```python
from build123d import *

# Parameters (mm, degrees)
F1_DEPTH = 25.4


with BuildPart() as f1:
    # F0 (on Front) → F1 (new body)
    with BuildSketch(Plane.XZ):
        Polygon((37.505187, 36.036089), (-59.895307, -2.682783), (38.255867, -41.096099), (18.550564, -2.999177), align=None)
        Polygon((5.644079, -12.203965), (-13.873555, -4.697184), (5.034152, -10.421105), align=None, mode=Mode.SUBTRACT)
        Polygon((11.606792, -2.682783), (26.432687, -31.33728), (-46.783395, -2.682783), (24.93133, 25.526594), (13.858826, 2.0679), (11.419123, 2.0679), (12.732809, 13.328073), (-28.366823, -2.682783), (13.1488, -18.930706), (7.523733, -8.055575), (-15.980633, -2.682783), align=None, mode=Mode.SUBTRACT)
        Polygon((6.774401, 3.053483), (-3.437838, 2.788078), (6.774401, 6.766378), align=None, mode=Mode.SUBTRACT)
    extrude(amount=F1_DEPTH)


solid = f1.part
```
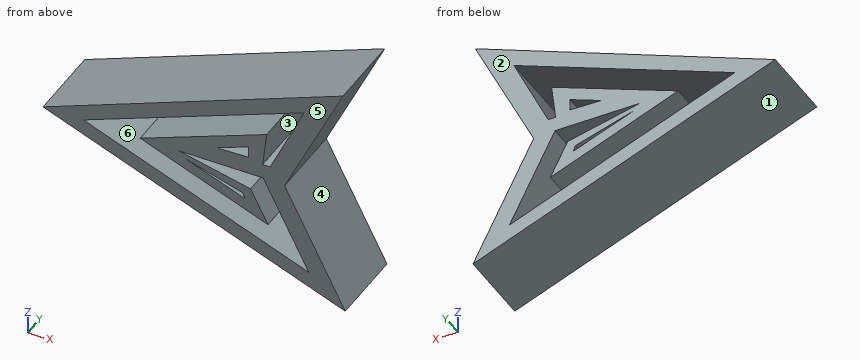
Input: part model. Units: mm. Frame: model coordinates. Face numbers are marked on the shaded views. A direction names the side the tool comes from. Coordinates: 2 decimals unless noted, no trailing zeros. Loops run counter-clockwise (first coordinate to the right, second up) from the corner with the lowest first, then second, coordinate; pieces in that order, holes last. Notation, with made-up numbers: M -25,29.5 L -13,29.5 A24 cw -13,58.5 Z; hole C -23.5,21 d8. An arc over 180 degrees is marked long. Answer in a Markdown table with one row per item.
1. Section D-D, the plane y = -11.75. Output: boundary loops of the cut face in (x, z), then the cut area to 3 significant figures.
Response:
| item | result |
|---|---|
| outline | M -59.9,-2.68 L 38.26,-41.1 L 18.55,-3 L 37.51,36.04 Z; hole M -46.78,-2.68 L 26.43,-31.34 L 11.61,-2.68 L -15.98,-2.68 L 7.52,-8.06 L 13.15,-18.93 L -28.37,-2.68 L 12.73,13.33 L 11.42,2.07 L 13.86,2.07 L 24.93,25.53 Z; hole M -13.87,-4.7 L 5.64,-12.2 L 5.03,-10.42 Z; hole M -3.44,2.79 L 6.77,3.05 L 6.77,6.77 Z |
| area | 1,870 mm2 |
2. Material intervals for line 1 (Z direction, x = -27, y = -2); line 2 (Z direction, x = 2, y = -16.25); line 3 (Z direction, x = 21.5, y = -6.25), sorted ascending.
Response:
| item | result |
|---|---|
| line 1 | z = -15.56 to -10.43, -3.22 to -2.15, 5.1 to 10.39 |
| line 2 | z = -26.91 to -21.78, -14.57 to -10.8, -9.5 to -6.79, -2.68 to 2.93, 4.91 to 9.15, 16.51 to 21.92 |
| line 3 | z = -34.54 to -29.41, -21.8 to -8.7, 3.07 to 18.26, 24.18 to 29.67 |
3. Section C-C, the plane x = -23.5. Output: boundary loops of the cut face in (y, z).
Response:
| item | result |
|---|---|
| outline | M -25.4,-16.93 L 0,-16.93 L 0,-11.8 L -25.4,-11.8 Z; M -25.4,-4.59 L 0,-4.59 L 0,-0.79 L -25.4,-0.79 Z; M -25.4,6.48 L 0,6.48 L 0,11.79 L -25.4,11.79 Z |
4. Section B-B, the plane z = 4.5. Output: boundary loops of the cut face in (x, y), then the cut area to 3 significant figures.
Response:
| item | result |
|---|---|
| outline | M -41.83,-25.4 L -28.52,-25.4 L -28.52,0 L -41.83,0 Z; M -9.93,-25.4 L 0.96,-25.4 L 0.96,0 L -9.93,0 Z; M 6.77,-25.4 L 11.7,-25.4 L 11.7,0 L 6.77,0 Z; M 15.01,-25.4 L 22.19,-25.4 L 22.19,0 L 15.01,0 Z |
| area | 922 mm2 |
5. Reachability of the marked faces 4, 5 and 6 from +Z, -Z, +X, -X, +Y, -Y: full face, straight path, thin tool, end or side. Return the list, or none.
Response:
| item | result |
|---|---|
| face 4 | +X, +Y, -Y |
| face 5 | +Z, -Z, +X, -X, -Y |
| face 6 | +Y, -Y |
6. Section A-A, the plane x = -42. Output: boundary loops of the cut face in (y, z).
Response:
| item | result |
|---|---|
| outline | M -25.4,-9.69 L 0,-9.69 L 0,-4.55 L -25.4,-4.55 Z; M -25.4,-0.8 L 0,-0.8 L 0,4.43 L -25.4,4.43 Z |
7. Draft query along Z for the marked faces 1, 2 and 3. Return one class per face: pulls with the +Z half, pulls with the -Z half, needs draft (parallel to the pull), parting line crosses it, or undercut.
Response:
| item | result |
|---|---|
| face 1 | pulls with the -Z half |
| face 2 | needs draft |
| face 3 | undercut |
8. First-contact query: pin 1 (2 mm diameter, centred on x = 12.5, y = -8, fed in from +Z); pin 2 (8 mm diameter, centred on x = 0, y = -18, fed in from +Z); pin 3 (2 mm diameter, centred on x = -24.5, y = -5.5, fed in from -Z). Flat tips, straight axial feed; report the tip coordinate or a pass-through.
Response:
| item | result |
|---|---|
| pin 1 | stops at z = 26.49 |
| pin 2 | stops at z = 22.72 |
| pin 3 | stops at z = -16.93 |
